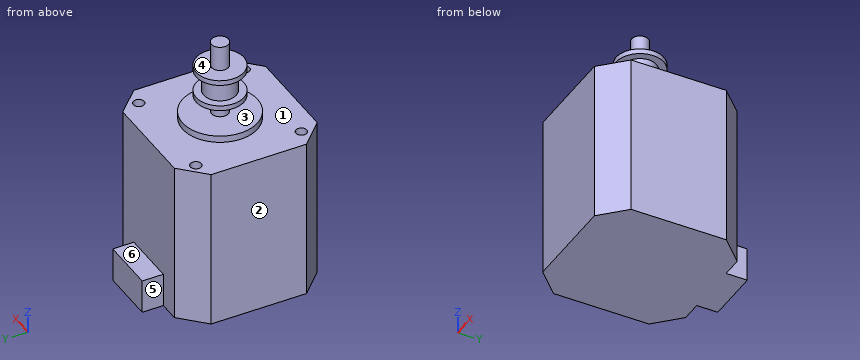
from build123d import *

# Parameters (mm, degrees)
SKETCH1_W           = 42
SKETCH1_H           = 42
BOSS_EXTRUDE1_DEPTH = 47.8
CHAMFER1_SIZE       = 7
SKETCH2_W           = 16
SKETCH2_H           = 6.2
BOSS_EXTRUDE2_DEPTH = 10
SKETCH3_R           = 11
BOSS_EXTRUDE3_DEPTH = 2
SKETCH4_R           = 1.6
CUT_EXTRUDE1_DEPTH  = 3


with BuildPart() as part:
    # Sketch1 → Boss-Extrude1 (new body)
    with BuildSketch(Plane.XY):
        with Locations((21, 21)):
            Rectangle(SKETCH1_W, SKETCH1_H)
    extrude(amount=BOSS_EXTRUDE1_DEPTH)

    # Chamfer1
    chamfer1_edges = [part.edges().sort_by_distance(p)[0] for p in [
        (0, 42, 23.9),
        (42, 42, 23.9),
        (42, 0, 23.9),
        (0, 0, 23.9),
    ]]
    chamfer(chamfer1_edges, length=CHAMFER1_SIZE)

    # Sketch2 → Boss-Extrude2 (add)
    with BuildSketch(Plane(origin=(0, 0, 0), x_dir=(-1, 0, 0), z_dir=(0, 0, -1))):
        with Locations((-21, 45.1)):
            Rectangle(SKETCH2_W, SKETCH2_H)
    extrude(amount=-BOSS_EXTRUDE2_DEPTH)

    # Sketch3 → Boss-Extrude3 (add)
    with BuildSketch(Plane.XY.offset(47.8)):
        with Locations((21, 21)):
            Circle(SKETCH3_R)
    extrude(amount=BOSS_EXTRUDE3_DEPTH)

    # Sketch4 → Cut-Extrude1 (cut)
    with BuildSketch(Plane.XY.offset(47.8)):
        with Locations((5.5, 36.5)):
            Circle(SKETCH4_R)
        with Locations((36.5, 36.5)):
            Circle(SKETCH4_R)
        with Locations((36.5, 5.5)):
            Circle(SKETCH4_R)
        with Locations((5.5, 5.5)):
            Circle(SKETCH4_R)
    extrude(amount=-CUT_EXTRUDE1_DEPTH, mode=Mode.SUBTRACT)

    # Sketch5 → Revolve1 (revolve)
    with BuildSketch(Plane(origin=(0, 21, 0), x_dir=(1, 0, 0), z_dir=(0, 1, 0)), mode=Mode.PRIVATE) as revolve1_sk:
        Polygon((23.5, -49.8), (21, -49.8), (21, -72), (23.5, -72), (23.5, -64.6), (28, -64.6), (28, -63.1), (25.8, -63.1), (25.8, -56.55), (28, -56.55), (28, -55.05), (23.5, -55.05), align=None)
    revolve(revolve1_sk.sketch.rotate(Axis((21, 21, 49.8), (0, 0, 1)), 180), axis=Axis((21, 21, 49.8), (0, 0, 1)))


solid = part.part
Verification items for the finished model (mm, model axes). Face numbers are marked on the shaded views. A direction names the side the tool comes from. Coordinates: 2 decimals unless noted, no trailing zeros. Order: outer loops, then holes, each group sorted by start corner. A loop starts at its lowest first (then second) coordinate and runs counter-clockwise, first axis right, second up. Notation, with made-up numbers: M 49,38.25 L 105,38.25 A21 cw 105,69.25 Z; hole C -29,-10 d4. An arc over 180 degrees is marked long. Write each question's results on one line, items separated by ' | '.
1) Access from +Z, -Z, +X, -X, +Y, -Y to the whole of each face (thin tool, end or side, straight path). Record for the marked faces 4, 5 and 6.
Solved:
face 4: +Z | face 5: +Z, -Z, -X, +Y | face 6: +Z, +X, -X, +Y
2) Release check for a two-part mould opening along Z. For the marked faces 1, 2 and 3 record: pulls with the +Z half, pulls with the -Z half, needs draft (parallel to the pull), parting line crosses it, or undercut.
Solved:
face 1: pulls with the +Z half | face 2: needs draft | face 3: undercut
3) Section check A-A on y = 36.5. Record the cut outline in (x, z).
Solved:
outline: M 1.5,0 L 40.5,0 L 40.5,47.8 L 38.1,47.8 L 38.1,44.8 L 34.9,44.8 L 34.9,47.8 L 7.1,47.8 L 7.1,44.8 L 3.9,44.8 L 3.9,47.8 L 1.5,47.8 Z
4) Section check D-D on y = 21. Record the cut outline in (x, z), plus the area to 3 significant figures.
Solved:
outline: M 0,0 L 42,0 L 42,47.8 L 32,47.8 L 32,49.8 L 23.5,49.8 L 23.5,55.05 L 28,55.05 L 28,56.55 L 25.8,56.55 L 25.8,63.1 L 28,63.1 L 28,64.6 L 23.5,64.6 L 23.5,72 L 18.5,72 L 18.5,64.6 L 14,64.6 L 14,63.1 L 16.2,63.1 L 16.2,56.55 L 14,56.55 L 14,55.05 L 18.5,55.05 L 18.5,49.8 L 10,49.8 L 10,47.8 L 0,47.8 Z | area: 2,220 mm²
5) Section check B-B on z = 32.5. Record the cut outline in (x, y).
Solved:
outline: M 0,7 L 7,0 L 35,0 L 42,7 L 42,35 L 35,42 L 7,42 L 0,35 Z
6) Gauge pin test, flat ends, axial feed: pin 1 Ø5 at (y, z) = (45.5, 4) entering from +X; pin 2 Ø3.5 at (x, y) = (37, 37) entering from +Z; pin 3 Ø5 at (y, z) = (44, 3) entering from -X. Record the tip position at first contact, or that the pin passes through.
Solved:
pin 1: stops at x = 29 | pin 2: stops at z = 47.8 | pin 3: stops at x = 6.5
7) Scan lines: line 1 along Y through (x, z) = (36.5, 46.8); line 2 along Y through (x, z) = (5, 45); line 3 along Z through (x, y) = (22, 37.5). Record each from-to range of solid material in increasing order. Write a range as [from, to].
Solved:
line 1: y = [1.5, 3.9], [7.1, 34.9], [38.1, 40.5] | line 2: y = [2, 3.98], [7.02, 34.98], [38.02, 40] | line 3: z = [0, 47.8]
